CAD build for the part. Positions are in the model's coordinates, mm. Face numbers are marked on the shaded views. A direction names the side the tool comes from. Give positions to 0.01 mm unless a question says otherwise; leave off trailing zeros. Loops run counter-clockwise (first coordinate to the right, second up) from the corner with the lowest first, then second, coordinate; pieces in that order, holes last. Notation, with made-up numbers: (76, 23) - (84, 23) arc R28 cw to (84, 62) - close; hole circle Ø8 at (84.5, -3.5). An arc over 180 degrees is marked (long way). Return JSON: item names as keys, results as strings.
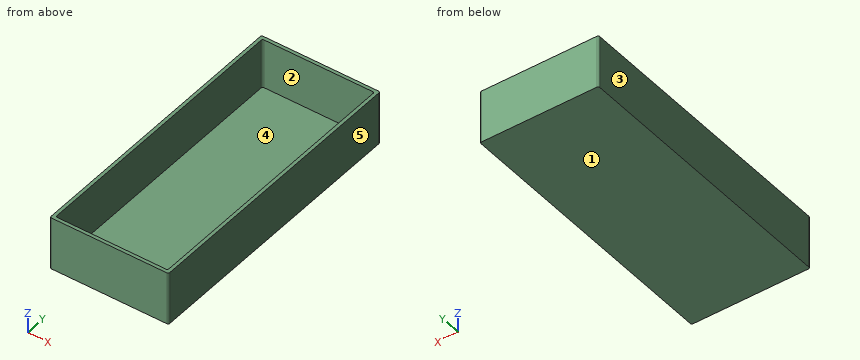
from build123d import *

# Parameters (mm, degrees)
F2_DEPTH = 40.64
F4_DEPTH = 38.1


# Not quite as in the source:
# - a variable given as a bare number and used for a length is read in inches; the dataset says mm whatever the document's units were


with BuildPart() as f2:
    # F1 (on Top) → F2 (new body)
    with BuildSketch(Plane.XY):
        with BuildLine():
            ThreePointArc((0, 1.27), (0.3719743879, 0.3719743879), (1.27, 0))
            Line((1.27, 0), (89.535, 0))
            ThreePointArc((89.535, 0), (90.4330256121, 0.3719743879), (90.805, 1.27))
            Line((90.805, 1.27), (90.805, 216.535))
            ThreePointArc((90.805, 216.535), (90.4330256121, 217.4330256121), (89.535, 217.805))
            Line((89.535, 217.805), (1.27, 217.805))
            ThreePointArc((1.27, 217.805), (0.3719743879, 217.4330256121), (0, 216.535))
            Line((0, 216.535), (0, 1.27))
        make_face()
    extrude(amount=F2_DEPTH)

    # F3 (on face) → F4 (cut)
    with BuildSketch(Plane.XY.offset(40.64)):
        with BuildLine():
            Line((2.54, 213.995), (2.54, 3.81))
            ThreePointArc((2.54, 3.81), (2.9119743879, 2.9119743879), (3.81, 2.54))
            Line((3.81, 2.54), (86.995, 2.54))
            ThreePointArc((86.995, 2.54), (87.8930256121, 2.9119743879), (88.265, 3.81))
            Line((88.265, 3.81), (88.265, 213.995))
            ThreePointArc((88.265, 213.995), (87.8930256121, 214.8930256121), (86.995, 215.265))
            Line((86.995, 215.265), (3.81, 215.265))
            ThreePointArc((3.81, 215.265), (2.9119743879, 214.8930256121), (2.54, 213.995))
        make_face()
    extrude(amount=-F4_DEPTH, mode=Mode.SUBTRACT)


solid = f2.part
1. Drill centre lines: probe 1 along Y at (x, z) = (86.5, 5.5) (3 decimals); probe 2 along X at (y, z) = (56.5, 20) (3 decimals); probe 3 along Z at (x, y) = (15, 152). Where is each one in solid material? Low to high.
Values follow:
{"probe 1": "y = 0 to 2.54, 215.265 to 217.805", "probe 2": "x = 0 to 2.54, 88.265 to 90.805", "probe 3": "z = 0 to 2.54"}
2. Pull direction X, two halves, no side cores. Call the marked faces 1, 2 and 3: +X half, -X half, draft (parallel to the pull), parting line (faces both ways), or undercut.
Values follow:
{"face 1": "draft", "face 2": "undercut", "face 3": "-X half"}
3. Cut at A-A, the plane z = 17. Write the cut outline in (x, y) (3 decimals), plus the area to 3 significant figures.
Values follow:
{"outline": "(0, 1.27) arc R1.27 ccw to (1.27, 0) - (89.535, 0) arc R1.27 ccw to (90.805, 1.27) - (90.805, 216.535) arc R1.27 ccw to (89.535, 217.805) - (1.27, 217.805) arc R1.27 ccw to (0, 216.535) - close; hole (2.54, 3.81) arc R1.27 ccw to (3.81, 2.54) - (86.995, 2.54) arc R1.27 ccw to (88.265, 3.81) - (88.265, 213.995) arc R1.27 ccw to (86.995, 215.265) - (3.81, 215.265) arc R1.27 ccw to (2.54, 213.995) - close", "area": "1,540 mm²"}
4. Drop a flat-ended pin along its axis: P1, Ø1.5, axis at x = 56, y = 55.5, coming from the +Z side. Give the stop position or say it passes through.
Values follow:
{"P1": "stops at z = 2.54"}
5. Cut at B-B, the plane x = 21. Write the cut outline in (y, z) (3 decimals), plus the area to 3 significant figures.
Values follow:
{"outline": "(0, 0) - (217.805, 0) - (217.805, 40.64) - (215.265, 40.64) - (215.265, 2.54) - (2.54, 2.54) - (2.54, 40.64) - (0, 40.64) - close", "area": "747 mm²"}
6. Which spindle directions (+Z, -Z, +X, -X, +Y, -Y) get a long thin tool onto all of the face, cutting with end or side? Do the marked faces 4 and 5. Say none if no direction does.
Values follow:
{"face 4": "+Z", "face 5": "+Z, -Z, +X, +Y, -Y"}
7. Cut at C-C, the plane y = 95.5. Write the cut outline in (x, z) (3 decimals).
Values follow:
{"outline": "(0, 0) - (90.805, 0) - (90.805, 40.64) - (88.265, 40.64) - (88.265, 2.54) - (2.54, 2.54) - (2.54, 40.64) - (0, 40.64) - close"}
